For this review, use the dimensioned drawing (mm, ordinates from the lowest corner) and the shaded views. A direction names the side the tool comes from. Round coordinates to 2 decimals unless told otherwise and drop trailing zeros. Loops run counter-clockwise (first coordinate to the right, second up) from the corner with the lowest first, then second, coordinate; pieces in that order, holes last. Notation, with made-up numbers: M 63.5,9 L 91.5,9 A31 cw 91.5,38 Z; hole C -3,-35.75 d10. An arc over 180 degrees is marked long. Use a Markdown table: item, result. Add a question column.
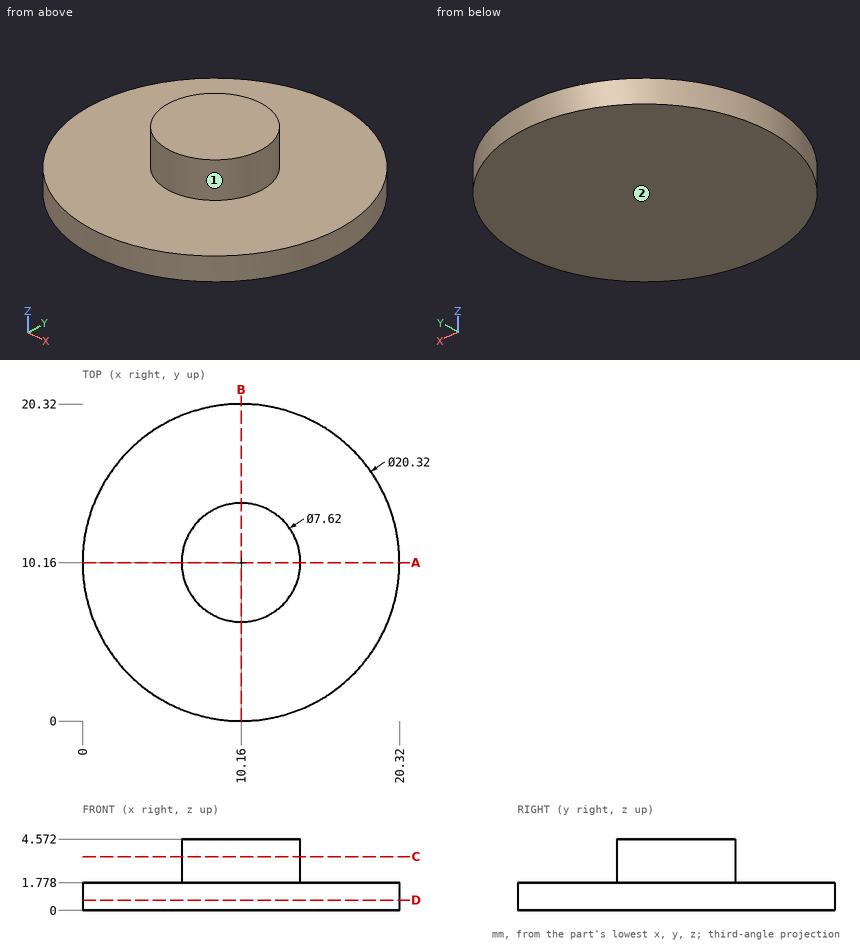
(1) Consider section C-C, the plane z = 3.45. Give the boundary of the cut face in (x, y).
(2) To check wall thickness, follow probe 1 along Z at (x, y) = (2.5, 16.5); probe 2 along X at (y, z) = (10.25, 0.9); probe 3 along X at (y, z) = (15, 1.6). State the ranges of each line that lie inside material, in increasing order.
(3) Consider section A-A, the plane y = 10.16. Give the boundary of the cut face in (x, z), then the cut area to 3 significant figures.
(4) For the marked faces 1 and 2, list the 3-axis set-ups (+Z, -Z, +X, -X, +Y, -Y) from which the entire face can be reached by the end or side of a thin tool; tool diameter is ignored.
(5) Consider section D-D, the plane z = 0.65. Give the boundary of the cut face in (x, y).
Found:
| question | item | result |
|---|---|---|
| 1 | outline | C 10.16,10.16 d7.62 |
| 2 | probe 1 | z = 0 to 1.78 |
| 2 | probe 2 | x = 0 to 20.32 |
| 2 | probe 3 | x = 1.23 to 19.09 |
| 3 | outline | M 0,0 L 20.32,0 L 20.32,1.78 L 13.97,1.78 L 13.97,4.57 L 6.35,4.57 L 6.35,1.78 L 0,1.78 Z |
| 3 | area | 57.4 mm^2 |
| 4 | face 1 | +Z |
| 4 | face 2 | -Z, +X, -X, +Y, -Y |
| 5 | outline | C 10.16,10.16 d20.32 |
